The listing builds one solid part. Answer for the finished solid, in the listing's coordinates (mm). A direction names the side the tool comes from. Round coordinates to 2 decimals unless told otherwise and drop trailing zeros. Write each loop counter-clockwise with the first axis right and the second up, starting at its lowest first coordinate (ties: lowest second). Pieces come first, ordered by that corner, then holes. Notation, with made-up numbers: M -7.5,68 L 10.5,68 A31 cw 10.5,102 Z; hole C 32,86.25 d7. An arc over 180 degrees is marked long. One line per item, written item: value. Start each with the question number.
(1) Section D-D (y = 16) is taken. Determine the outline of the cut face in (x, z), plus the area to 3 significant figures.
(2) Consider probe 1 along Y at (x, z) = (-1.55, -9.9); probe 2 along Y at (x, z) = (-2.1, 9.9); probe 3 along Y at (x, z) = (-8.75, 3.5). Determine where each line is inside the solid, lowest interval first.
(3) Section A-A (y = 23.65) is taken. Determine the outline of the cut face in (x, z), plus the area to 3 significant figures.
(4) Section B-B (z = 9.9) is taken. Determine the outline of the cut face in (x, y).
(5) For faces 4 (the flat face through (-2, 24, -14)), 5 (the flat face through (-8, -11, 0)), 6 (the flat face through (-2, 20, 7.1)), 7 (the flat face through (-2, 9, -7.1)), 8 (the cylindrical face through (-6.386, 34.423, 0.477)), determine the directions among +Z, -Z, +X, -X, +Y, -Y from which every point of the face is accessible in a straight line to the end or side of a thin tool.
(6) For a pull along X with two mould halves and no side action, classify faces 1 (the cylindrical face through (-6.386, -5.423, -0.477)), 2 (the cylindrical face through (-10.922, 14.297, -6.425)), 3 (the cylindrical face through (-1.58, 22.65, -8.59)) as released by +X, released by -X, zero draft, split by the parting line, or undercut.
(7) Given P1, Ø1.5, axis at x = -6, z = -2, coming from the +Y side; P2, Ø1, axis at x = -1.5, y = 16.5, coming from the +Z side; P3, Ø1, axis at x = -1, z = -9, coming from the -Y side; P4, Ø4.5, axis at y = 14.5, z = 11, coming from the -X side, each flat-ended and moving along its own axis, determine where each tip first touches the part or whether it passes through.
(8) Section C-C (x = -7.9) is taken. Determine the outline of the cut face in (y, z).
Autodesk Inventor part; units mm, degrees
ref_plane "YZ Plane" through (0, 0, 0) normal (1, 0, 0) x (0, 1, 0)
ref_plane "XZ Plane" through (0, 0, 0) normal (0, 1, 0) x (-1, 0, 0)
ref_plane "XY Plane" through (0, 0, 0) normal (0, 0, 1) x (1, 0, 0)
sketch "Sketch1" plane through (0, 0, 0) normal (0, 1, 0) x (-1, 0, 0)
  arc A0 (3.2, -5.3217) -> (15, 0) centre (7.9, 0) ccw
  line L0 (3.2, -5.3217) -> (3.2, -14)
  line L1 (3.2, -14) -> (0, -14)
  line L2 (0, -14) -> (0, 14)
  line L3 (0, 14) -> (3.2, 14)
  line L4 (3.2, 14) -> (3.2, 5.3217)
  arc A1 (15, 0) -> (3.2, 5.3217) centre (7.9, 0) ccw
  line L5 (7.9, 7.1) -> (7.9, -7.1) construction
  line L6 (3.2, 5.3217) -> (15, 0) construction
  line L7 (3.2, -5.3217) -> (15, 0) construction
  point P0 (0, 0)
  point P1 (0, 0)
  dimension "d0" = 3.2
  dimension "d1" = 28
  dimension "d5" = 14.2
  dimension "d6" = 15
extrude "Extrusion1" add sketch "Sketch1" along normal blind 29
sketch "Sketch2" plane through (0, 0, 14) normal (1, 0, 0) x (0, 0, -1)
  circle A0 centre (23.9, 23.65) radius 1.65
  circle A1 centre (4.1, 5.35) radius 1.65
  line L0 (23.9, 23.65) -> (23.9, 5.35) construction
  line L1 (23.9, 5.35) -> (4.1, 5.35) construction
  line L2 (28, 0) -> (28, 29)
  line L3 (0, 0) -> (0, 29)
  line L4 (23.9, 23.65) -> (28, 23.65) construction
  line L5 (23.9, 23.65) -> (28, 29) construction
  line L6 (0, 0) -> (4.1, 5.35) construction
  line L7 (4.1, 5.35) -> (0, 5.35) construction
  line L8 (28, 18.3) -> (21.1, 18.3)
  line L9 (21.1, 18.3) -> (21.1, 0)
  line L10 (21.1, 0) -> (28, 0)
  line L11 (0, 10.7) -> (6.9, 10.7)
  line L12 (6.9, 10.7) -> (6.9, 29)
  line L13 (6.9, 29) -> (0, 29)
  line L14 (28, 18.3) -> (23.9, 23.65) construction
  point P0 (14, 0)
  dimension "d9" = 19.8
  dimension "d10" = 18.3
  dimension "d11" = 3.3
  dimension "d12" = 2.8
extrude "Extrusion2" cut sketch "Sketch2" against normal up to surface (3.2 mm away)
sketch "Sketch3" plane through (0, 0, 0) normal (0, -1, 0) x (1, 0, 0)
  arc A0 (-3.2, 5.3217) -> (-3.2, -5.3217) centre (-7.9, 0) ccw
  circle A1 centre (-7.9, 0) radius 1.5875
  point P0 (0, 0)
  dimension "d15" = 3.175
extrude "Extrusion3" add sketch "Sketch3" along normal blind 11
sketch "Sketch4" plane through (0, 29, 0) normal (0, 1, 0) x (1, 0, 0)
  arc A0 (-3.2, 5.3217) -> (-3.2, -5.3217) centre (-7.9, 0) ccw construction
  circle A1 centre (-7.9, 0) radius 1.5875
  point P0 (0, 0)
  dimension "d18" = 3.175
extrude "Extrusion4" add sketch "Sketch4" along normal blind 11
properties part number "Power Resistor - HSA25" material "Gold"
Recorded:
1. outline: M -15,0 A7.1 ccw -3.2,-5.32 L -3.2,-7.1 L 0,-7.1 L 0,7.1 L -3.2,7.1 L -3.2,5.32 A7.1 ccw Z
1. area: 186 mm2
2. probe 1: y = 18.3 to 22, 25.3 to 29
2. probe 2: y = 0 to 3.7, 7 to 10.7
2. probe 3: y = 0 to 29
3. outline: M -15,0 A7.1 ccw -3.2,-5.32 L -3.2,-8.25 L 0,-8.25 L 0,7.1 L -3.2,7.1 L -3.2,5.32 A7.1 ccw Z; M -3.2,-14 L 0,-14 L 0,-11.55 L -3.2,-11.55 Z
3. area: 198 mm2
4. outline: M -3.2,0 L 0,0 L 0,3.7 L -3.2,3.7 Z; M -3.2,7 L 0,7 L 0,10.7 L -3.2,10.7 Z
5. face 4: -Z, +X, -X, +Y, -Y
5. face 5: +Z, -Z, +X, -X, -Y
5. face 6: +Z, +X, -X, +Y
5. face 7: -Z, +X, -X, -Y
5. face 8: +Y
6. face 1: split by the parting line
6. face 2: undercut
6. face 3: zero draft
7. P1: stops at y = 29
7. P2: stops at z = 7.1
7. P3: stops at y = 18.3
7. P4: passes through
8. outline: M -11,-1.59 L 0,-1.59 L 0,-7.1 L 29,-7.1 L 29,-1.59 L 40,-1.59 L 40,1.59 L 29,1.59 L 29,7.1 L 0,7.1 L 0,1.59 L -11,1.59 Z
